Part model, mm, in its own coordinate system. A direction names the side the tool comes from. Round coordinates to 2 decimals unless told otherwise and drop trailing zeros. Loops run counter-clockwise (first coordinate to the right, second up) from the corner with the lowest first, then second, coordinate; pieces in that order, holes last.
1) Band-saw the part on C-C, the plane x = 0.5. Write the cut outline in (y, z), then the cut area to 3 significant figures.
2) Mould opens along Y. For faces 5 (the flat face through (-9, 1, 3.2)), 6 (the flat face through (11.802, 33.807, 1.578)), 7 (the flat face through (18.01, -0.84, 0.79)) say: +Y half, -Y half, draft (parallel to the pull), parting line (faces both ways), or undercut.
3) Probe line 1 (Y direction, x = -15.5, z = 0.3); line 2 (X direction, y = 2.5, z = 1.45); line 3 (X direction, y = -2, z = 0.2). List the from-to ranges inside material, lowest first.
4) Band-saw the part on A-A, the plane z = 1. State how many separate pieces and enclosed holes the cut face has, then the cut area to 3 significant figures.
5) 3-axis set-ups, long thin cutter, end or side, ignore diameter. For faces 1 (the flat face through (8.72, 5.69, 2.39)), 2 (the flat face through (-16.54, -31.74, 1.58)), 3 (the flat face through (-1, 1, 0)), 4 (the flat face through (-20, 7.675, 2)): which of +Z, -Z, +X, -X, +Y, -Y reach the whole face in a straight line?
6) Drop flat-ended pins along their axis: P1, Ø1.3, axis at x = 14, z = 1, coming from the +Y side; P2, Ø0.5, axis at x = 15.5, z = 1, coming from the -Y side; P3, Ø1, axis at x = -17, z = 2.5, coming from the -Y side; P4, Ø3, axis at x = 3, y = 19, coming from the -Z side. Give the stop position or say it passes through.
7) Band-saw the part on B-B, the plane y = -27.5. Write the cut outline in (x, z), then the cut area to 3 significant figures.
from build123d import *

# Parameters (mm, degrees)
F1_DEPTH = 3.2
F2_DEPTH = 1.6
F3_DEPTH = 2.5


# Not quite as in the source:
# - a feature names something its author has since deleted; it is built from what else it names


with BuildPart() as f1:
    # F0 (on Top) → F1 (new body)
    with BuildSketch(Plane.XY):
        with BuildLine():
            Line((-12.0286401361, 7.7058477327), (2.8731075212, 24.026809333))
            ThreePointArc((2.8731075212, 24.026809333), (-23.1446184854, 7.061795007), (-11.0294978873, -21.5381635686))
            Line((-11.0294978873, -21.5381635686), (-4.3697794008, -9.2094279826))
            Line((-4.3697794008, -9.2094279826), (-18.230907619, -9.2094279826))
            Line((-18.230907619, -9.2094279826), (-2.0674222615, 7.7058477327))
            Line((-2.0674222615, 7.7058477327), (-12.0286401361, 7.7058477327))
        make_face()
        with BuildLine():
            add(Edge.make_bspline(
                [(-14.0679626526, 6.3070743063), (-12.6996164354, 4.9387280892), (-12.6996164354, 2.4824249728)],
                knots=[0, 0, 0, 1, 1, 1], degree=2))
            add(Edge.make_bspline(
                [(-12.6996164354, 2.4824249728), (-12.6996164354, -0.138404107), (-14.1224184292, -1.5252884609)],
                knots=[0, 0, 0, 1, 1, 1], degree=2))
            add(Edge.make_bspline(
                [(-14.1224184292, -1.5252884609), (-15.545220423, -2.9121728148), (-18.2170293788, -2.9121728148)],
                knots=[0, 0, 0, 1, 1, 1], degree=2))
            Line((-18.2170293788, -2.9121728148), (-21.1506895159, -2.9121728148))
            Line((-21.1506895159, -2.9121728148), (-21.1506895159, 7.6754205235))
            Line((-21.1506895159, 7.6754205235), (-17.9065155886, 7.6754205235))
            add(Edge.make_bspline(
                [(-17.9065155886, 7.6754205235), (-15.4363088697, 7.6754205235), (-14.0679626526, 6.3070743063)],
                knots=[0, 0, 0, 1, 1, 1], degree=2))
        make_face(mode=Mode.SUBTRACT)
        with BuildLine():
            ThreePointArc((-11.0294978873, -21.5381635686), (-23.1446184854, 7.061795007), (2.8731075212, 24.026809333))
            Line((2.8731075212, 24.026809333), (4.1858882241, 25.464616759))
            ThreePointArc((4.1858882241, 25.464616759), (-24.5061657926, 8.0880285022), (-11.7940875977, -22.9536024329))
            Line((-11.7940875977, -22.9536024329), (-11.0294978873, -21.5381635686))
        make_face()
        Polygon((4.1858882241, 25.464616759), (2.8731075212, 24.026809333), (-12.0286401361, 7.7058477327), (-2.0674222615, 7.7058477327), (-18.230907619, -9.2094279826), (-4.3697794008, -9.2094279826), (-11.0294978873, -21.5381635686), (-11.7940875977, -22.9536024329), (-21.4260146022, -40.7846085727), (-7.468564605, -24.7020021385), (-6.3056047528, -23.3619704275), (10.7070716166, -3.7589499261), (1.6710584512, -3.7589499261), (15.9755367786, 15.4116954654), (5.7308066454, 15.4116954654), (9.2615315623, 22.3554545173), (9.9925901152, 23.7932030147), (19.2086462315, 41.9181135037), align=None)
    extrude(amount=F1_DEPTH)

    # F0 (on Top) → F2 (join)
    with BuildSketch(Plane.XY):
        with BuildLine():
            ThreePointArc((-6.3056047528, -23.3619704275), (22.9064425811, -7.7998206282), (9.2615315623, 22.3554545173))
            Line((9.2615315623, 22.3554545173), (5.7308066454, 15.4116954654))
            Line((5.7308066454, 15.4116954654), (15.9755367786, 15.4116954654))
            Line((15.9755367786, 15.4116954654), (1.6710584512, -3.7589499261))
            Line((1.6710584512, -3.7589499261), (10.7070716166, -3.7589499261))
            Line((10.7070716166, -3.7589499261), (-6.3056047528, -23.3619704275))
        make_face()
        with BuildLine():
            Line((16.7712777882, 1.29050713), (14.6610901855, 1.29050713))
            Line((14.6610901855, 1.29050713), (14.6610901855, -2.912172582))
            Line((14.6610901855, -2.912172582), (13.4865518028, -2.912172582))
            Line((13.4865518028, -2.912172582), (13.4865518028, 7.1941661569))
            Line((13.4865518028, 7.1941661569), (16.258108476, 7.1941661569))
            add(Edge.make_bspline(
                [(16.258108476, 7.1941661569), (18.1183472327, 7.1941661569), (19.0064398139, 6.4819225426)],
                knots=[0, 0, 0, 1, 1, 1], degree=2))
            add(Edge.make_bspline(
                [(19.0064398139, 6.4819225426), (19.8945323952, 5.7696789282), (19.8945323952, 4.3385558895)],
                knots=[0, 0, 0, 1, 1, 1], degree=2))
            add(Edge.make_bspline(
                [(19.8945323952, 4.3385558895), (19.8945323952, 2.3345412479), (17.8617625766, 1.6289334436)],
                knots=[0, 0, 0, 1, 1, 1], degree=2))
            Line((17.8617625766, 1.6289334436), (20.6067760095, -2.912172582))
            Line((20.6067760095, -2.912172582), (19.2176797679, -2.912172582))
            Line((19.2176797679, -2.912172582), (16.7712777882, 1.29050713))
        make_face(mode=Mode.SUBTRACT)
        with BuildLine():
            Line((-12.0286401361, 7.7058477327), (2.8731075212, 24.026809333))
            ThreePointArc((2.8731075212, 24.026809333), (-23.1446184854, 7.061795007), (-11.0294978873, -21.5381635686))
            Line((-11.0294978873, -21.5381635686), (-4.3697794008, -9.2094279826))
            Line((-4.3697794008, -9.2094279826), (-18.230907619, -9.2094279826))
            Line((-18.230907619, -9.2094279826), (-2.0674222615, 7.7058477327))
            Line((-2.0674222615, 7.7058477327), (-12.0286401361, 7.7058477327))
        make_face()
        with BuildLine():
            add(Edge.make_bspline(
                [(-14.0679626526, 6.3070743063), (-12.6996164354, 4.9387280892), (-12.6996164354, 2.4824249728)],
                knots=[0, 0, 0, 1, 1, 1], degree=2))
            add(Edge.make_bspline(
                [(-12.6996164354, 2.4824249728), (-12.6996164354, -0.138404107), (-14.1224184292, -1.5252884609)],
                knots=[0, 0, 0, 1, 1, 1], degree=2))
            add(Edge.make_bspline(
                [(-14.1224184292, -1.5252884609), (-15.545220423, -2.9121728148), (-18.2170293788, -2.9121728148)],
                knots=[0, 0, 0, 1, 1, 1], degree=2))
            Line((-18.2170293788, -2.9121728148), (-21.1506895159, -2.9121728148))
            Line((-21.1506895159, -2.9121728148), (-21.1506895159, 7.6754205235))
            Line((-21.1506895159, 7.6754205235), (-17.9065155886, 7.6754205235))
            add(Edge.make_bspline(
                [(-17.9065155886, 7.6754205235), (-15.4363088697, 7.6754205235), (-14.0679626526, 6.3070743063)],
                knots=[0, 0, 0, 1, 1, 1], degree=2))
        make_face(mode=Mode.SUBTRACT)
    extrude(amount=F2_DEPTH)

    # F0 (on Top) → F3 (join)
    with BuildSketch(Plane.XY):
        with BuildLine():
            ThreePointArc((-11.0294978873, -21.5381635686), (-23.1446184854, 7.061795007), (2.8731075212, 24.026809333))
            Line((2.8731075212, 24.026809333), (4.1858882241, 25.464616759))
            ThreePointArc((4.1858882241, 25.464616759), (-24.5061657926, 8.0880285022), (-11.7940875977, -22.9536024329))
            Line((-11.7940875977, -22.9536024329), (-11.0294978873, -21.5381635686))
        make_face()
    extrude(amount=F3_DEPTH)


solid = f1.part
Reported:
1. outline: (-24.19, 0) - (25.8, 0) - (25.8, 3.2) - (-15.52, 3.2) - (-15.52, 1.6) - (-24.19, 1.6) - close
1. area: 146 mm2
2. face 5: draft
2. face 6: +Y half
2. face 7: undercut
3. line 1: y = -33.96 to -29.81, -20.63 to -2.43, 7.25 to 20.63
3. line 2: x = -25.68 to -21.15, -12.7 to 13.49, 19.26 to 24.07
3. line 3: x = -25.73 to -21.15, -14.7 to 13.49, 14.66 to 18.69, 20.06 to 24.12
4. separate pieces: 1
4. enclosed holes: 2
4. area: 1,950 mm2
5. face 1: +Z, +X
5. face 2: +Z, -Z, -X
5. face 3: -Z, +X, -X, +Y, -Y
5. face 4: +Z, -Z
6. P1: stops at y = 36.93
6. P2: stops at y = -18.79
6. P3: stops at y = -36.26
6. P4: stops at z = 0
7. outline: (-14.25, 0) - (-9.9, 0) - (-9.9, 3.2) - (-14.25, 3.2) - close
7. area: 13.9 mm2
